```python
from build123d import *

# Parameters (mm, degrees)
CROQUIS1_W              = 100
CROQUIS1_H              = 20
SALIENTE_EXTRUIR1_DEPTH = 10
CORTAR_EXTRUIR1_DEPTH   = 52.961524227
MATRIZL1_COUNT          = 69
MATRIZL1_PITCH          = 4.71


with BuildPart() as part:
    # Croquis1 → Saliente-Extruir1 (new body)
    with BuildSketch(Plane.XY):
        Rectangle(CROQUIS1_W, CROQUIS1_H)
    extrude(amount=SALIENTE_EXTRUIR1_DEPTH)

    # Croquis2 → Cortar-Extruir1 (cut, through all)
    with BuildSketch(Plane.XY.offset(10)):
        Polygon((-43.275, 10), (-44.375, 6.75), (-45.625, 6.75), (-46.725, 10), align=None)
    cortar_extruir1 = extrude(amount=-CORTAR_EXTRUIR1_DEPTH, mode=Mode.SUBTRACT)

    # MatrizL1: Cortar-Extruir1 ×69
    with Locations(*[(i * MATRIZL1_PITCH, 0, 0) for i in range(1, MATRIZL1_COUNT)]):
        add(cortar_extruir1, mode=Mode.SUBTRACT)


solid = part.part
```
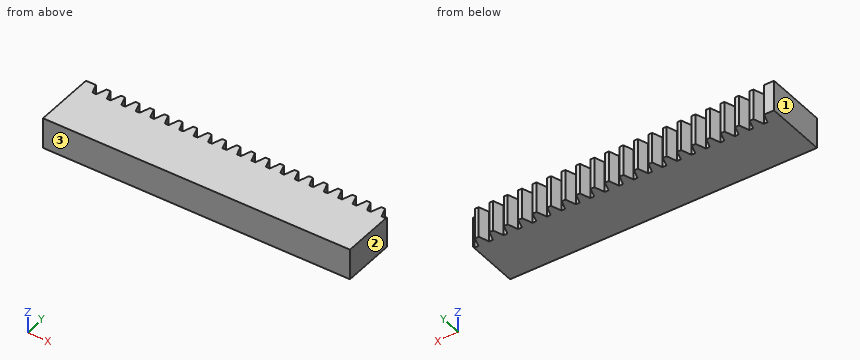
The model under review builds one solid part; all positions refer to its coordinate system, in mm. Face numbers are marked on the shaded views. Round coordinates to 2 decimals unless told otherwise and drop trailing zeros. Use a Markdown table: item, result.
1) Insertion check: pin 1 (0.6 mm diameter, centred on x = -7.5, z = 4, fed in from +Y). The pin has a flat end and moves straight along its axis. Give the tip position at first contact, or say it passes through.
Report:
| item | result |
|---|---|
| pin 1 | y = 6.75 |
2) Consider section A-A (y = 8.25). Give the number of separate pieces and of enclosed holes in the cut face, then the cut area to 3 significant figures.
Report:
| item | result |
|---|---|
| separate pieces | 21 |
| enclosed holes | 0 |
| area | 528 mm^2 |
3) Wall thickness on line 1 along Y through (x, z) = (-44.5, 7.25): over which ranges is the line inside the solid? List them lowest first. Write a range as [from, to].
Report:
| item | result |
|---|---|
| line 1 | [-10, 6.75] |
4) Draft analysis for pull direction X (two halves, no side actions). For the marked faces 1, 2 and 3, state which applies: released by +X, released by -X, zero draft, split by the parting line, or undercut.
Report:
| item | result |
|---|---|
| face 1 | released by -X |
| face 2 | released by +X |
| face 3 | zero draft |
